Verification items for this drawing (mm, ordinates from the low corner). A direction names the side the tool comes from. Give positions to 0.01 mm unless a question says otherwise; leave off trailing zeros. Loops run counter-clockwise (first coordinate to the right, second up) from the corner with the lowest first, then second, coordinate; pieces in that order, holes last. Notation, with made-up numbers: (-18, 5.25) -> (7, 5.25) arc R18 cw to (7, 34.25) -> close; hole circle Ø9 at (80, -12.75). An arc over 180 degrees is marked (long way). Answer as a JSON object with one key per item and string values.
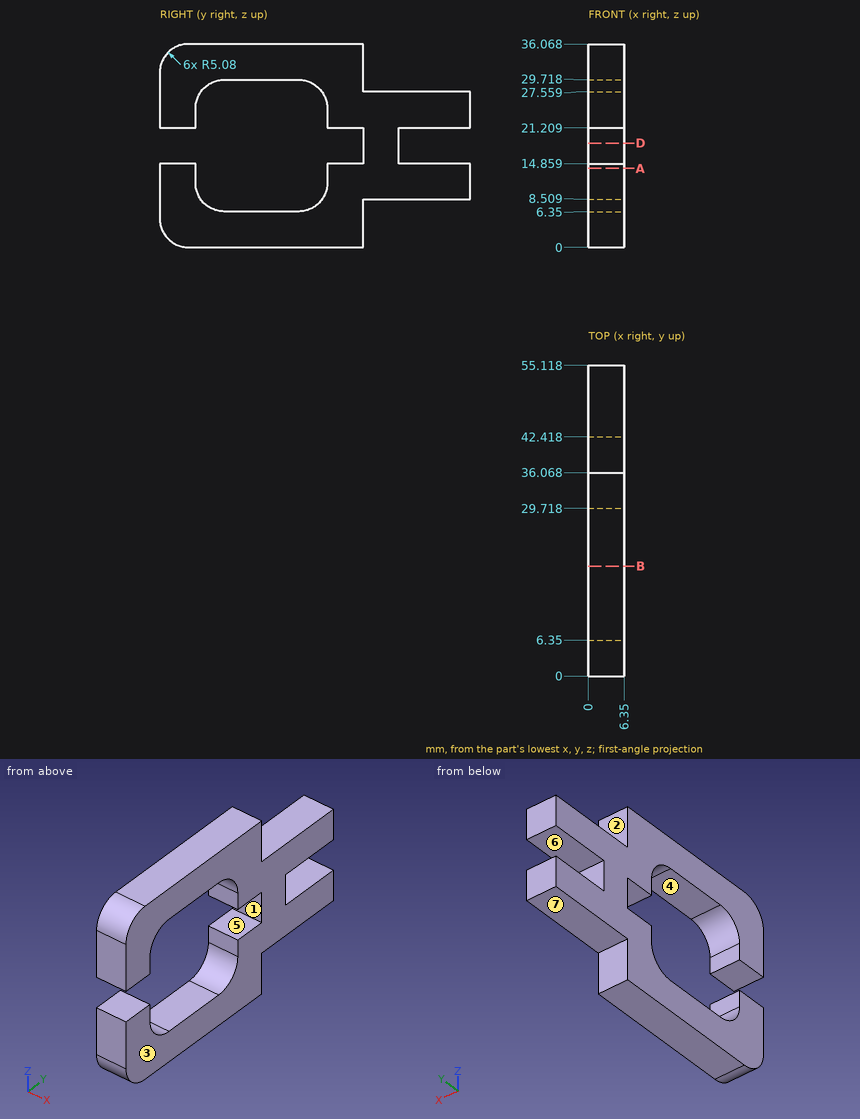
1) Material ranges on line 1 along Z through (x, y) = (0.5, 50); line 2 along Y through (x, z) = (5.5, 12.5); line 3 along Z through (x, y) = (4.75, 17), recorded low to high. Write a range as from..to.
Geometry check:
{"line 1": "z = 8.51..14.86, 21.21..27.56", "line 2": "y = 0..6.35, 29.72..55.12", "line 3": "z = 0..6.35, 29.72..36.07"}
2) Section check B-B on y = 19.5. Record the cut outline in (x, z).
Geometry check:
{"outline": "(0, 0) -> (6.35, 0) -> (6.35, 6.35) -> (0, 6.35) -> close; (0, 29.72) -> (6.35, 29.72) -> (6.35, 36.07) -> (0, 36.07) -> close"}
3) Depth check by flat-ended pin: P1, Ø1.9, axis at x = 2, z = 18.5, coming from the -Y side; P2, Ø1, axis at y = 48.5, z = 6.5, coming from the -X side; P3, Ø1.9, axis at x = 4.5, y = 44.5, coming from the -Z side; P4, Ø1.5, axis at x = 3.5, z = 30, coming from the +Y side. Enter the tip coordinate at first touch or a pass-through.
Geometry check:
{"P1": "stops at y = 36.07", "P2": "passes through", "P3": "stops at z = 8.51", "P4": "stops at y = 36.07"}
4) Section check D-D on z = 18.5. Record the cut outline in (x, y).
Geometry check:
{"outline": "(0, 36.07) -> (6.35, 36.07) -> (6.35, 42.42) -> (0, 42.42) -> close"}
5) Tool access check on the marked faces 5, 6 and 7. Record the directions out of +Z, -Z, +X, -X, +Y, -Y that give a thin tool (end or side, any length) a straight path to the whole face; none if there is none.
Geometry check:
{"face 5": "+X, -X, -Y", "face 6": "+X, -X, +Y", "face 7": "-Z, +X, -X, +Y"}
6) Section check A-A on z = 14. Record the cut outline in (x, y).
Geometry check:
{"outline": "(0, 0) -> (6.35, 0) -> (6.35, 6.35) -> (0, 6.35) -> close; (0, 29.72) -> (6.35, 29.72) -> (6.35, 55.12) -> (0, 55.12) -> close"}
7) Draft check along Y on the marked faces 1, 2, 3 and 4. Enter one of: pulls with the +Y half, pulls with the -Y half, needs draft (parallel to the pull), parting line crosses it, or undercut.
Geometry check:
{"face 1": "pulls with the -Y half", "face 2": "pulls with the +Y half", "face 3": "needs draft", "face 4": "undercut"}
